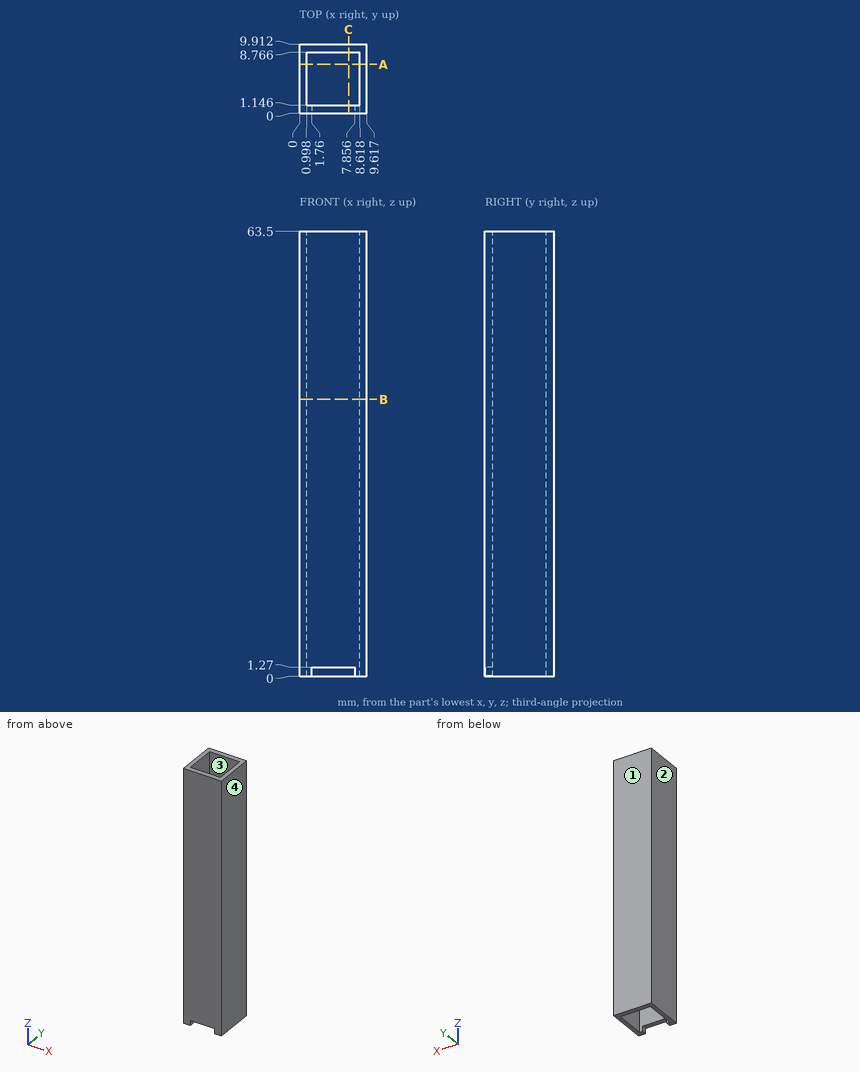
Answer from the drawing. Dimensions are ordinates in mm from the lowest x, y and z of the part. Coordinates: 2 decimals unless noted, no trailing zeros. Write each loop counter-clockwise with the first axis right and the second up, starting at its lowest first coordinate (ties: lowest second). Pieces come first, ordered by that corner, then holes. Notation, with made-up numbers: (14.5, 42) - (61.5, 42) arc R25 cw to (61.5, 59) - close; hole circle Ø4 at (-17, 39.25). An arc over 180 degrees is marked (long way). Return JSON: item names as keys, results as strings. Group by question number.
Q1. A flat-ended cylindrical pin translates along its axis: pin 1 Ø0.6 at (x, y) = (3.5, 0.5) entering from -Z. Find the tip coordinate at first contact, or state that the pin passes through.
Q2. The part is cut by section B-B on z = 39.5. Write down the section's boundary in (x, y).
Q3. Find the intervals of material crossed by line 1 along X through (y, z) = (6.25, 31); line 2 along Y through (x, z) = (5.25, 45), in increasing order. Write a range as [from, to].
Q4. For a pull along X with two mould halves and no side action, classify the marked faces 1, 2, 3 and 4 as +X half, -X half, draft (parallel to the pull), parting line (faces both ways), or undercut.
Q5. The part is cut by section A-A on y = 7. Write down the section's boundary in (x, z), and give its area (3 significant figures).
Q6. The part is cut by section C-C on x = 7. Write down the section's boundary in (y, z), and give its area (3 significant figures).
Evaluation:
{
 "1": {"pin 1": "stops at z = 1.27"},
 "2": {"outline": "(0, 0) - (9.62, 0) - (9.62, 9.91) - (0, 9.91) - close; hole (1, 1.15) - (8.62, 1.15) - (8.62, 8.77) - (1, 8.77) - close"},
 "3": {"line 1": "x = [0, 1], [8.62, 9.62]", "line 2": "y = [0, 1.15], [8.77, 9.91]"},
 "4": {"face 1": "draft", "face 2": "-X half", "face 3": "undercut", "face 4": "+X half"},
 "5": {"outline": "(0, 0) - (1, 0) - (1, 63.5) - (0, 63.5) - close; (8.62, 0) - (9.62, 0) - (9.62, 63.5) - (8.62, 63.5) - close", "area": "127 mm2"},
 "6": {"outline": "(0, 1.27) - (1.15, 1.27) - (1.15, 63.5) - (0, 63.5) - close; (8.77, 0) - (9.91, 0) - (9.91, 63.5) - (8.77, 63.5) - close", "area": "144 mm2"}
}
